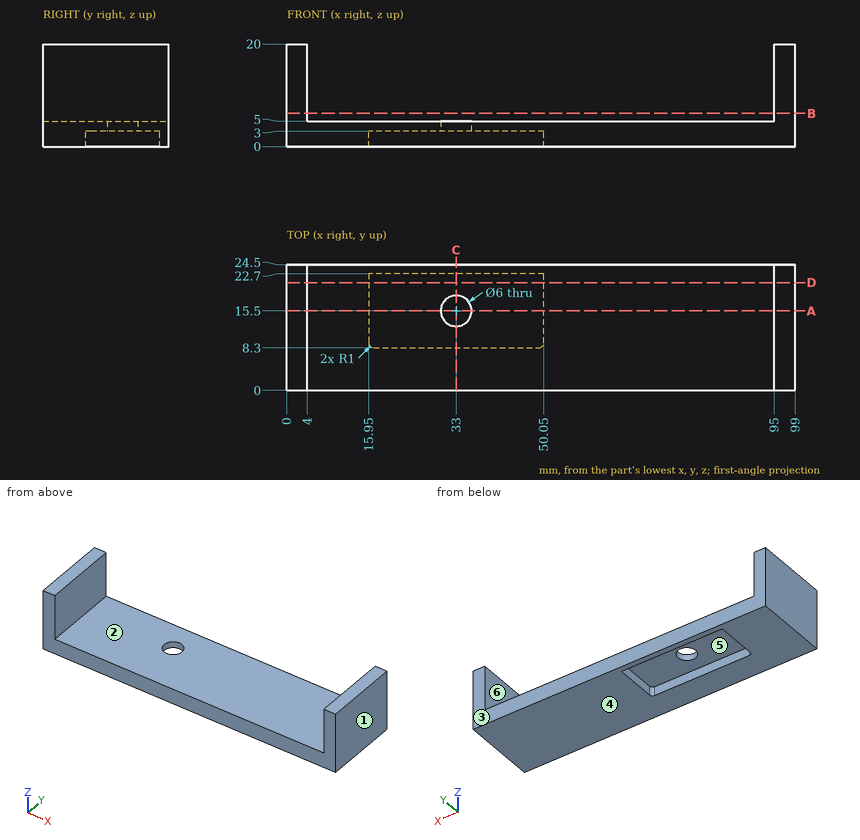
Geometry check sheet. Reference: drawing and pictorial views, mm from the part's lowest x, y, z. A direction names the side the tool comes from. Coordinates: 2 decimals unless noted, no trailing zeros. Order: outer loops, then holes, each group sorted by start corner. A loop starts at its lowest first (then second) coordinate and runs counter-clockwise, first axis right, second up. Notation, with made-up numbers: (11, -29) -> (18, -29) arc R29 ccw to (18, 4) -> close; hole circle Ø4 at (53.25, -24). An arc over 180 degrees is marked (long way). Put each result on its own line as item: value. Start each with the question number.
1) Release check for a two-part mould opening along X. For the marked faces 1, 2 and 3 record: pulls with the +X half, pulls with the -X half, needs draft (parallel to the pull), parting line crosses it, or undercut.
2) Tool access check on the marked faces 4, 5 and 6. Record the directions out of +Z, -Z, +X, -X, +Y, -Y that give a thin tool (end or side, any length) a straight path to the whole face; none if there is none.
3) Cross-section at C-C (x = 33). Enter the section's corners in (y, z).
4) Go/stop test with flat-tipped pins: pin 1 (7.5 mm diameter, centred on x = 68, y = 9, fed in from +Z); pin 2 (6 mm diameter, centred on x = 39.5, z = 8.5, fed in from -Y). Record where each tip stops, or that it passes through.
5) Cross-section at D-D (y = 21). Enter the section's corners in (x, z).
6) Material ranges on L1, parallel to X at y = 3.75, z = 10.5; L2, parallel to Y at x = 33, z = 3.8; L3, parallel to Z at x = 48.5, y = 7.5, recorded low to high.
7) Cross-section at A-A (y = 15.5). Enter the section's corners in (x, z).
8) Cross-section at B-B (z = 6.5). Enter the section's corners in (x, y).
Geometry check:
1. face 1: pulls with the +X half
1. face 2: undercut
1. face 3: needs draft
2. face 4: -Z, +X, -X, +Y, -Y
2. face 5: -Z
2. face 6: +Z, +Y, -Y
3. outline: (0, 0) -> (8.3, 0) -> (8.3, 3) -> (12.5, 3) -> (12.5, 5) -> (0, 5) -> close; (18.5, 3) -> (22.7, 3) -> (22.7, 0) -> (24.5, 0) -> (24.5, 5) -> (18.5, 5) -> close
4. pin 1: stops at z = 5
4. pin 2: passes through
5. outline: (0, 0) -> (15.95, 0) -> (15.95, 3) -> (50.05, 3) -> (50.05, 0) -> (99, 0) -> (99, 20) -> (95, 20) -> (95, 5) -> (4, 5) -> (4, 20) -> (0, 20) -> close
6. L1: x = 0 to 4, 95 to 99
6. L2: y = 0 to 12.5, 18.5 to 24.5
6. L3: z = 0 to 5
7. outline: (0, 0) -> (15.95, 0) -> (15.95, 3) -> (30, 3) -> (30, 5) -> (4, 5) -> (4, 20) -> (0, 20) -> close; (36, 3) -> (50.05, 3) -> (50.05, 0) -> (99, 0) -> (99, 20) -> (95, 20) -> (95, 5) -> (36, 5) -> close
8. outline: (0, 0) -> (4, 0) -> (4, 24.5) -> (0, 24.5) -> close; (95, 0) -> (99, 0) -> (99, 24.5) -> (95, 24.5) -> close
